```python
from build123d import *

# Parameters (mm, degrees)
CYLINDER004_R     = 1.5
CYLINDER004_DEPTH = 3
CYLINDER003_R     = 3.8
CYLINDER003_DEPTH = 2.1
CYLINDER002_R     = 4
CYLINDER002_DEPTH = 2.5


with BuildPart() as cylinder004:
    # Cylinder004 → Cylinder004 (new body)
    with BuildSketch(Plane.XY):
        Circle(CYLINDER004_R)
    extrude(amount=CYLINDER004_DEPTH)


with BuildPart() as fusion:
    # Cylinder003 → Cylinder003 (new body)
    with BuildSketch(Plane.XY):
        Circle(CYLINDER003_R)
    extrude(amount=CYLINDER003_DEPTH)

    # Fusion: union Cylinder004
    add(cylinder004.part)


with BuildPart() as cut001:
    # Cylinder002 → Cylinder002 (new body)
    with BuildSketch(Plane.XY):
        Circle(CYLINDER002_R)
    extrude(amount=CYLINDER002_DEPTH)

    # Cut001: cut Fusion
    add(fusion.part, mode=Mode.SUBTRACT)


solid = cut001.part
```
Input: part model. Units: mm. Frame: model coordinates. A direction names the side the tool comes from. Coordinates: 2 decimals unless noted, no trailing zeros. Order: outer loops, then holes, each group sorted by start corner. A loop starts at its lowest first (then second) coordinate and runs counter-clockwise, first axis right, second up. Notation, with made-up numbers: (27.25, -16.75) - (42.25, -16.75) arc R26 ccw to (42.25, 18.25) - close; hole circle Ø8 at (36.5, 28). An arc over 180 degrees is marked (long way). Return JSON: item names as keys, results as strings.
Q1. Cut plane B-B (y = -1.25). Return loops of the section in (x, z), then the cut area to 3 significant figures.
The answers:
{"outline": "(-3.8, 0) - (-3.59, 0) - (-3.59, 2.1) - (-0.83, 2.1) - (-0.83, 2.5) - (-3.8, 2.5) - close; (0.83, 2.1) - (3.59, 2.1) - (3.59, 0) - (3.8, 0) - (3.8, 2.5) - (0.83, 2.5) - close", "area": "3.26 mm2"}
Q2. First-contact query: pin 1 (1.5 mm diameter, centred on x = -1, z = 2, fed in from -Y); pin 2 (4 mm diameter, centred on x = 0, y = 0, fed in from -Z); pin 3 (1.5 mm diameter, centred on x = -2, z = 2, fed in from +Y). Flat tips, straight axial feed; report the tip coordinate or a pass-through.
The answers:
{"pin 1": "stops at y = -3.99", "pin 2": "stops at z = 2.1", "pin 3": "stops at y = 3.8"}
Q3. Cut plane C-C (z = 1.75). Return loops of the section in (x, y), then the cut area to 3 significant figures.
The answers:
{"outline": "circle Ø8 at (0, 0); hole circle Ø7.6 at (0, 0)", "area": "4.90 mm2"}
Q4. Cut plane A-A (x = 0). Return loops of the section in (y, z), then the cut area to 3 significant figures.
The answers:
{"outline": "(-4, 0) - (-3.8, 0) - (-3.8, 2.1) - (-1.5, 2.1) - (-1.5, 2.5) - (-4, 2.5) - close; (1.5, 2.1) - (3.8, 2.1) - (3.8, 0) - (4, 0) - (4, 2.5) - (1.5, 2.5) - close", "area": "2.84 mm2"}
Q5. Access query for faces 4 (the cylindrical face through (-1.5, 0.07, 2.3)), 5 (the cylindrical face through (-3.796, 0.167, 1.035)). Directions: +Z, -Z, +X, -X, +Y, -Y. A direction counts if a zero-diameter tool reaches every point of the face in a straight line with its end or side. Return the directions, or none.
The answers:
{"face 4": "+Z, -Z", "face 5": "-Z"}
Q6. Ray query, probe 1 along Y at (x, z) = (0, 2.35); probe 2 along Y at (x, z) = (0, 1.25); probe 3 along Z at (x, y) = (1.25, -2). Return the intervals inside material, ascending.
The answers:
{"probe 1": "y = -4 to -1.5, 1.5 to 4", "probe 2": "y = -4 to -3.8, 3.8 to 4", "probe 3": "z = 2.1 to 2.5"}
Q7. Cut plane D-D (x = 3.25). Return loops of the section in (y, z), then the cut area to 3 significant figures.
The answers:
{"outline": "(-2.33, 0) - (-1.97, 0) - (-1.97, 2.1) - (1.97, 2.1) - (1.97, 0) - (2.33, 0) - (2.33, 2.5) - (-2.33, 2.5) - close", "area": "3.39 mm2"}
Q8. Draft query along X for faces 1 (the flat face through (2, 0, 2.5)), 2 (the flat face through (2, 0, 2.1)), 3 (the cylindrical face through (-0.867, -3.905, 1.232)). Return one class per face: +X half, -X half, draft (parallel to the pull), parting line (faces both ways), or undercut.
The answers:
{"face 1": "draft", "face 2": "undercut", "face 3": "parting line"}
